Input: part model. Units: mm. Frame: model coordinates. A direction names the side the tool comes from. Coordinates: 2 decimals unless noted, no trailing zeros. Order: outer loops, then holes, each group sorted by start corner. A loop starts at its lowest first (then second) coordinate and runs counter-clockwise, first axis right, second up. Notation, with made-up numbers: M 14.5,67.25 L 29.5,67.25 A25 ccw 29.5,91.25 Z; hole C 75,5 d3. An arc over 180 degrees is marked long. Answer in a Markdown table with one row per item.
Autodesk Inventor part; units mm, degrees
ref_plane "YZ Plane" through (0, 0, 0) normal (1, 0, 0) x (0, 1, 0)
ref_plane "XZ Plane" through (0, 0, 0) normal (0, 1, 0) x (-1, 0, 0)
ref_plane "XY Plane" through (0, 0, 0) normal (0, 0, 1) x (1, 0, 0)
sketch "Szkic1" plane through (0, 0, 0) normal (0, 0, 1) x (1, 0, 0)
  line L0 (72, -75) -> (-72, -75)
  line L1 (-72, -75) -> (-72, 75)
  line L2 (-72, 75) -> (72, 75)
  line L3 (72, 75) -> (72, -75)
  line L4 (72, -75) -> (-72, 75) construction
  line L5 (-72, -75) -> (72, 75) construction
  point P0 (0, 0)
  dimension "d0" = 144
  dimension "d1" = 150
extrude "Wyciągnięcie proste1" add sketch "Szkic1" along normal blind 3
sketch "Szkic2" plane through (0, 0, 3) normal (0, 0, 1) x (1, 0, 0)
  line L0 (72, -75) -> (72, 75)
  line L1 (-72, -75) -> (72, -75)
  line L2 (72, -75) -> (72, 75)
  line L3 (72, 75) -> (-72, 75)
  line L4 (-72, 75) -> (-72, -75)
  line L5 (-72, -75) -> (72, 75) construction
  line L6 (72, -75) -> (-72, 75) construction
  line L7 (-20, 17.5) -> (20, 17.5)
  line L8 (20, 17.5) -> (20, 57.5)
  line L9 (20, 57.5) -> (-20, 57.5)
  line L10 (-20, 57.5) -> (-20, 17.5)
  point P0 (0, 0)
  point P1 (53.5, -2.5)
  point P2 (53.5, -51.5)
  point P3 (-4.5, -51.5)
  point P4 (-4.5, -2.5)
  dimension "d12" = 58
  dimension "d14" = 58
  dimension "d15" = 49
  dimension "d16" = 18.5
  dimension "d17" = 72.5
  dimension "d18" = 23.5
  dimension "d19" = 18.5
  dimension "d20" = 23.5
  dimension "d21" = 40
  dimension "d22" = 40
  dimension "d23" = 20
  dimension "d24" = 52
hole "Otwór1" at (53.5, -2.5, 3) at (53.5, -51.5, 3) at (-4.5, -51.5, 3) at (-4.5, -2.5, 3) at (-20, 57.5, 3) at (20, 57.5, 3) at (20, 17.5, 3) at (-20, 17.5, 3) direction (0, 0, -1) diameter 3 end through all
sketch "Szkic3" plane through (0, 0, 3) normal (0, 0, 1) x (1, 0, 0)
  line L0 (-30, 67.5) -> (-10, 67.5)
  line L1 (-10, 75) -> (-10, 7.5)
  line L2 (-10, 7.5) -> (-30, 7.5)
  line L3 (-30, 7.5) -> (-30, 75)
  circle A0 centre (-20, 57.5) radius 1.5
  line L4 (10, 67.5) -> (30, 67.5)
  line L5 (30, 67.5) -> (30, 0)
  line L6 (30, 0) -> (10, 0)
  line L7 (10, 0) -> (10, 67.5)
  circle A1 centre (20, 57.5) radius 1.5
  line L8 (30, 67.5) -> (30, 47.5)
  line L9 (-30, 47.5) -> (-30, 67.5)
  line L10 (-14.5, 7.5) -> (5.5, 7.5)
  line L11 (5.5, 7.5) -> (5.5, -61.5)
  line L12 (5.5, -61.5) -> (-14.5, -61.5)
  line L13 (-14.5, -61.5) -> (-14.5, 7.5)
  circle A2 centre (-4.5, -51.5) radius 1.5
  circle A3 centre (-4.5, -2.5) radius 1.5
  line L14 (-30, 67.5) -> (30, 67.5)
  line L15 (30, 67.5) -> (30, 47.5)
  line L16 (30, 47.5) -> (-30, 47.5)
  line L17 (-30, 47.5) -> (-30, 67.5)
  line L18 (-14.5, 7.5) -> (63.5, 7.5)
  line L19 (63.5, 7.5) -> (63.5, -12.5)
  line L20 (63.5, -12.5) -> (-14.5, -12.5)
  line L21 (-14.5, -12.5) -> (-14.5, 7.5)
  circle A4 centre (53.5, -2.5) radius 1.5
  line L22 (63.5, 7.5) -> (43.5, 7.5)
  line L23 (43.5, 7.5) -> (43.5, -61.5)
  line L24 (43.5, -61.5) -> (63.5, -61.5)
  line L25 (63.5, -61.5) -> (63.5, 7.5)
  circle A5 centre (53.5, -51.5) radius 1.5
  line L26 (-14.5, -61.5) -> (63.5, -61.5)
  line L27 (63.5, -61.5) -> (63.5, -41.5)
  line L28 (63.5, -41.5) -> (-14.5, -41.5)
  line L29 (-14.5, -41.5) -> (-14.5, -61.5)
  line L30 (72, 75) -> (-72, 75)
  line L31 (-72, -75) -> (72, -75)
  line L32 (-72, 75) -> (72, 75)
  line L33 (72, 75) -> (72, -75)
  line L34 (72, -75) -> (-72, -75)
  line L35 (-72, -75) -> (-72, 75)
  line L36 (-30, 67.5) -> (-10, 67.5)
  line L37 (-10, 67.5) -> (-10, 7.5)
  line L38 (-10, 7.5) -> (-30, 7.5)
  line L39 (-30, 7.5) -> (-30, 67.5)
  point P0 (0, 0)
  dimension "d32" = 20
  dimension "d33" = 10
  dimension "d34" = 20
  dimension "d36" = 10
  dimension "d37" = 20
  dimension "d39" = 20
  dimension "d40" = 10
  dimension "d42" = 10
  dimension "d44" = 10
  dimension "d46" = 10
  dimension "d47" = 10
  dimension "d48" = 60
  dimension "d49" = 20
  dimension "d51" = 78
  dimension "d52" = 10
  dimension "d53" = 20
  dimension "d54" = 20
  dimension "d55" = 78
  dimension "d56" = 20
extrude "Wyciągnięcie proste2" cut sketch "Szkic3" against normal blind 10 contours L3 L30 L1 L0 | L3 L2 L13 L12 L26 L24 L25 L19 L18 L5 L4 L14 L1 L30 L33 L31 L35 | L16 L7 L18 L10 L1 | L20 L23 L28 L11
sketch "Szkic4" plane through (0, 0, 3) normal (0, 0, 1) x (1, 0, 0)
  line L0 (30, 7.5) -> (30, 67.5)
  line L1 (63.5, 7.5) -> (63.5, -61.5)
  line L2 (30, 67.5) -> (63.5, 7.5)
  line L3 (30, 7.5) -> (63.5, 7.5)
  line L4 (63.5, 7.5) -> (30, 7.5)
  line L5 (-30, 67.5) -> (30, 67.5)
  line L6 (30, 7.5) -> (30, 67.5)
  line L7 (-19, -71.5) -> (1, -71.5)
  line L8 (1, -71.5) -> (1, -61.5)
  line L9 (1, -61.5) -> (-19, -61.5)
  line L10 (-19, -61.5) -> (-19, -71.5)
  line L11 (-19, -71.5) -> (1, -61.5) construction
  line L12 (1, -71.5) -> (-19, -61.5) construction
  circle A0 centre (-4.5, -51.5) radius 1.5
  line L13 (-19, -61.5) -> (-14.5, -61.5)
  line L14 (-30, 7.5) -> (-30, 67.5)
  line L15 (63.5, -12.5) -> (72, -12.5)
  line L16 (72, -12.5) -> (72, 7.5)
  line L17 (72, 7.5) -> (63.5, 7.5)
  line L18 (63.5, 7.5) -> (63.5, -12.5)
  line L19 (63.5, -12.5) -> (72, 7.5) construction
  line L20 (72, -12.5) -> (63.5, 7.5) construction
  circle A1 centre (53.5, -2.5) radius 1.5
  line L21 (-14.5, -61.5) -> (-14.5, 7.5)
  line L22 (-14.5, 7.5) -> (-72, 7.5)
  line L23 (-72, 7.5) -> (-72, -12.5)
  line L24 (-72, -12.5) -> (-14.5, -12.5)
  line L25 (-14.5, -12.5) -> (-14.5, 7.5)
  line L26 (-72, -12.5) -> (-19, -61.5)
  line L27 (-14.5, -61.5) -> (-14.5, -12.5)
  point P0 (0, 0)
  point P1 (-9, -66.5)
  point P2 (67.75, -2.5)
  dimension "d59" = 20
  dimension "d60" = 10
  dimension "d61" = 15
  dimension "d62" = 4.5
  dimension "d63" = 8.5
  dimension "d64" = 20
  dimension "d65" = 18.5
  dimension "d67" = 10
  dimension "d68" = 57.5
  dimension "d69" = 20
extrude "Wyciągnięcie proste3" add sketch "Szkic4" against normal blind 3 contours L22 L21 L24 L23 | L17 L16 L15 L1 | L0 L2 L3 | L21 L9 L26 L24 | L9 L8 L7 L10
sketch "Szkic5" plane through (0, 0, 3) normal (0, 0, 1) x (1, 0, 0)
  line L0 (63.5, 7.5) -> (72, 7.5)
  line L1 (72, 7.5) -> (68, 7.5)
  line L2 (68, 7.5) -> (68, -12.5)
  line L3 (68, -12.5) -> (72, -12.5)
  line L4 (72, -12.5) -> (72, 7.5)
  line L5 (-72, 7.5) -> (-30, 7.5)
  line L6 (-72, 7.5) -> (-68, 7.5)
  line L7 (-68, 7.5) -> (-68, -12.5)
  line L8 (-68, -12.5) -> (-72, -12.5)
  line L9 (-72, -12.5) -> (-72, 7.5)
  line L10 (1, -71.5) -> (-19, -71.5)
  line L11 (1, -61.5) -> (1, -71.5)
  line L12 (-19, -71.5) -> (1, -71.5)
  line L13 (1, -71.5) -> (1, -67.5)
  line L14 (1, -67.5) -> (-19, -67.5)
  line L15 (-19, -67.5) -> (-19, -71.5)
  point P0 (0, 0)
  dimension "d72" = 4
  dimension "d73" = 20
  dimension "d74" = 4
  dimension "d75" = 4
extrude "Wyciągnięcie proste4" add sketch "Szkic5" along normal blind 10
sketch "Szkic6" plane through (-72, -12.5, 0) normal (-1, 0, 0) x (0, 0, 1)
  line L0 (13, 0) -> (13, 20)
  line L1 (0, 20) -> (13, 20)
  point P0 (0, 12.5)
  point P1 (8, 10)
  dimension "d78" = 5
  dimension "d79" = 10
hole "Otwór2" at (-72, -2.5, 8) direction (1, 0, 0) diameter 3 end through all
sketch "Szkic7" plane through (-19, -67.5, 3) normal (0, 1, 0) x (1, 0, 0)
  line L0 (20, -10) -> (0, -10)
  line L1 (20, 0) -> (20, -10)
  point P0 (19, 3)
  point P1 (10, -5)
  dimension "d87" = 5
  dimension "d88" = 10
hole "Otwór3" at (-9, -67.5, 8) direction (0, -1, 0) diameter 3 end through all
sketch "Szkic8" plane through (0, 0, 3) normal (0, 0, 1) x (1, 0, 0)
  line L0 (-72, -12.5) -> (-19, -61.5)
  line L1 (-19.1082, -54.5905) -> (-19.1082, 2.5)
  line L2 (-19.1082, 2.5) -> (-62.5745, 2.5)
  line L3 (-72, 7.5) -> (-30, 7.5)
  line L4 (-62.5745, 2.5) -> (-62.5745, -14.4046)
  line L5 (-62.5745, -14.4046) -> (-19.1082, -54.5905)
  line L6 (-72, 7.5) -> (-72, -12.5)
  line L7 (63.5, 7.5) -> (30, 67.5)
  line L8 (30, 57.8154) -> (30, 2.5)
  line L9 (30, 57.8154) -> (60.8845, 2.5)
  line L10 (30, 2.5) -> (60.8845, 2.5)
  line L11 (-30, 67.5) -> (-30, 7.5)
  point P0 (0, 0)
  dimension "d97" = 5
  dimension "d98" = 16.9046
  dimension "d99" = 40.1859
  dimension "d100" = 9.4254
  dimension "d102" = 5
  dimension "d103" = 55.3154
  dimension "d104" = 60
extrude "Wyciągnięcie proste5" cut sketch "Szkic8" against normal blind 10
properties part number "Uchwyt_elektronika"
1) Material intervals for probe 1 along Y at (x, z) = (-4.5, 0.9); probe 2 along X at (y, z) = (1.5, 4.25); probe 3 along X at (y, z) = (-2.5, 1.5), sorted ascending.
Resolved:
| item | result |
|---|---|
| probe 1 | y = -71.5 to -53, -50 to -4, -1 to 7.5, 47.5 to 67.5 |
| probe 2 | x = -72 to -68, 68 to 72 |
| probe 3 | x = -72 to -62.57, -19.11 to -6, -3 to 52, 55 to 72 |
2) Reachability of faces 4 (the face through (70, -12.5, 5)), 5 (the face through (68, -5, 8)), 6 (the face through (70, 7.5, 5)), 7 (the face through (-70, -12.5, 8)) from +Z, -Z, +X, -X, +Y, -Y: full face, straight path, thin tool, end or side. Return the list, or none.
Resolved:
| item | result |
|---|---|
| face 4 | +Z, -Z, +X, -Y |
| face 5 | +Z, +Y, -Y |
| face 6 | +Z, -Z, +X, +Y |
| face 7 | +Z, +X, -X, -Y |
3) Cut plane B-B, the plane y = 42. Output: boundary loops of the cut face in (x, z).
Resolved:
| item | result |
|---|---|
| outline | M -30,0 L -10,0 L -10,3 L -30,3 Z; M 10,0 L 30,0 L 30,3 L 10,3 Z; M 38.83,0 L 44.24,0 L 44.24,3 L 38.83,3 Z |
4) Mould query, pull axis X, two halves, no side actions, for faces 1 (the face through (-19, -69, 5)), 2 (the face through (13, 1, 3)), 3 (the face through (-11, -67.5, 8)). Classes: +X half, -X half, draft (parallel to the pull), parting line (faces both ways), or undercut.
Resolved:
| item | result |
|---|---|
| face 1 | -X half |
| face 2 | undercut |
| face 3 | draft |
5) Contact query for flat-ended pins moving along their axis: pin 1 (2.5 mm diameter, centred on x = 46, z = 2, fed in from +Y); pin 2 (2 mm diameter, centred on y = 41.5, z = 2.5, fed in from -X); pin 3 (8 mm diameter, centred on x = 21, y = -36, fed in from +Z); pin 4 (4.5 mm diameter, centred on x = -69.5, z = 8.5, fed in from -Y). Output: stop coordinate, or through.
Resolved:
| item | result |
|---|---|
| pin 1 | stops at y = 41.08 |
| pin 2 | stops at x = -30 |
| pin 3 | passes through |
| pin 4 | stops at y = -12.5 |
6) Cut plane A-A, the plane y = -10. Output: boundary loops of the cut face in (x, z), and give its area (3 significant figures).
Resolved:
| item | result |
|---|---|
| outline | M -72,0 L -62.57,0 L -62.57,3 L -68,3 L -68,13 L -72,13 Z; M -19.11,0 L 72,0 L 72,13 L 68,13 L 68,3 L -19.11,3 Z |
| area | 382 mm2 |
7) Cut plane C-C, the plane x = 41. Output: boundary loops of the cut face in (y, z), and give its area (3 significant figures).
Resolved:
| item | result |
|---|---|
| outline | M -61.5,0 L -41.5,0 L -41.5,3 L -61.5,3 Z; M -12.5,0 L 2.5,0 L 2.5,3 L -12.5,3 Z; M 38.11,0 L 47.8,0 L 47.8,3 L 38.11,3 Z |
| area | 134 mm2 |
